```python
from build123d import *

# Parameters (mm, degrees)
F1_DEPTH = 10.16
F0_R     = 26.4895980544
F2_DEPTH = 50.8
F3_W     = 45.2943015844
F3_H     = 10.4296095669
F4_DEPTH = 40.64
F6_DEPTH = 41.5868318139


with BuildPart() as f1:
    # F0 (on Top) → F1 (new body)
    with BuildSketch(Plane.XY):
        with BuildLine():
            Line((-38.4405590594, 29.9478769302), (-38.4405590594, -29.9478769302))
            Line((-38.4405590594, -29.9478769302), (38.4405590594, -29.9478769302))
            Line((38.4405590594, -29.9478769302), (38.4405590594, -29.5841870222))
            ThreePointArc((38.4405590594, -29.5841870222), (23.2267408591, 0), (38.4405590594, 29.5841870222))
            Line((38.4405590594, 29.5841870222), (38.4405590594, 29.9478769302))
            Line((38.4405590594, 29.9478769302), (-38.4405590594, 29.9478769302))
        make_face()
    extrude(amount=F1_DEPTH)

    # F0 (on Top) → F2 (join)
    with BuildSketch(Plane.XY):
        with BuildLine():
            ThreePointArc((38.4405590594, 29.5841870222), (23.2267408591, 0), (38.4405590594, -29.5841870222))
            ThreePointArc((38.4405590594, -29.5841870222), (76.2312009837, -32.3447137991), (95.9687949199, 0))
            ThreePointArc((95.9687949199, 0), (76.2312009837, 32.3447137991), (38.4405590594, 29.5841870222))
        make_face()
        with Locations((59.5977678895, 0)):
            Circle(F0_R, mode=Mode.SUBTRACT)
    extrude(amount=F2_DEPTH)

    # F3 (on face) → F4 (join)
    with BuildSketch(Plane.XY.offset(10.16)):
        with Locations((2.1366886795, 0)):
            Rectangle(F3_W, F3_H)
    extrude(amount=F4_DEPTH)

    # F5 (on face) → F6 (cut, through all)
    with BuildSketch(Plane.XZ.offset(5.2148047835)):
        Polygon((-20.5104621127, 50.8), (-20.5104621127, 10.16), (23.6025262829, 50.8), align=None)
    extrude(amount=-F6_DEPTH, mode=Mode.SUBTRACT)


solid = f1.part
```
Geometry: final body of the model. Coordinates: model frame, mm. A direction names the side the tool comes from. Round coordinates to 2 decimals unless told otherwise and drop trailing zeros. Order: outer loops, then holes, each group sorted by start corner. A loop starts at its lowest first (then second) coordinate and runs counter-clockwise, first axis right, second up. Notation, with made-up numbers: (49.5, 0) -> (58.5, 0) arc R19 cw to (58.5, 19) -> close; hole circle Ø7 at (-0.75, 58). An arc over 180 degrees is marked (long way). Use one line per item in the form item = value. Start each with the question number.
1. Reachability of faces 1 (the face through (1, 29.948, 5)), 2 (the face through (11, 5.215, 21)), 3 (the face through (-1, -29.948, 5)), 4 (the face through (-9, 7, 10.16)) from +Z, -Z, +X, -X, +Y, -Y: full face, straight path, thin tool, end or side. Return the list, or none.
2. Pin query (flat end, axial travel): pin 1 Ø1.5 at (x, y) = (79, -15) entering from -Z; pin 2 Ø12 at (x, z) = (9, 35) entering from +Y; pin 3 Ø10 at (x, z) = (76, 25) entering from +Y; pin 4 Ø12 at (y, z) = (4.5, 10) entering from +X. Return the tip coordinate at first contact, or that it passes through.
3. Cut plane D-D (y = 17). Return the cut outline in (x, z).
4. Line query: probe 1 along Z at (x, y) = (-28, -22); probe 2 along X at (y, z) = (17, 40.5); probe 3 along X at (y, z) = (-3.5, 22.5). Output: solid intervals per line, ascending.
5. Cut plane C-C (x = 48.5). Return the cut outline in (y, z), then the cut area to 3 significant figures.
6. Cut plane B-B (z = 6.5). Return the cut outline in (x, y).
7. Cut plane A-A (y = 0). Return the cut outline in (x, z).
8. Draft query along X for faces 5 (the face through (11, -5.215, 21)), 6 (the face through (1.24, -0.07, 30.2)), 7 (the face through (84.864, 7.957, 25.044)). Return one class per face: pulls with the +X half, pulls with the -X half, needs draft (parallel to the pull), parting line crosses it, or undercut.
Solution:
q1.face_1 = +Z, -Z, -X, +Y
q1.face_2 = +Z, -X, +Y
q1.face_3 = +Z, -Z, -X, -Y
q1.face_4 = +Z, -X
q2.pin_1 = through
q2.pin_2 = 5.21
q2.pin_3 = 34.54
q2.pin_4 = 95.97
q3.outline = (-38.44, 0) -> (39.28, 0) -> (39.28, 50.8) -> (27.44, 50.8) -> (27.44, 10.16) -> (-38.44, 10.16) -> close; (79.91, 0) -> (91.75, 0) -> (91.75, 50.8) -> (79.91, 50.8) -> close
q4.probe_1 = 0 to 10.16
q4.probe_2 = 27.44 to 39.28, 79.91 to 91.75
q4.probe_3 = -7.12 to 33.34, 85.86 to 95.8
q5.outline = (-34.64, 0) -> (-24.05, 0) -> (-24.05, 50.8) -> (-34.64, 50.8) -> close; (24.05, 0) -> (34.64, 0) -> (34.64, 50.8) -> (24.05, 50.8) -> close
q5.area = 1,080 mm^2
q6.outline = (-38.44, -29.95) -> (38.44, -29.95) -> (38.44, -29.58) arc R36.37 ccw (long way) to (38.44, 29.58) -> (38.44, 29.95) -> (-38.44, 29.95) -> close; hole circle Ø52.98 at (59.6, 0)
q7.outline = (-38.44, 0) -> (33.11, 0) -> (33.11, 50.8) -> (23.6, 50.8) -> (-20.51, 10.16) -> (-38.44, 10.16) -> close; (86.09, 0) -> (95.97, 0) -> (95.97, 50.8) -> (86.09, 50.8) -> close
q8.face_5 = needs draft
q8.face_6 = pulls with the -X half
q8.face_7 = undercut
